Autodesk Fusion 360 part; units mm, degrees
box "Primitiva de caixa1" add length 60 width 30 height 5 placed x (0, 1, 0) y (-1, 0, 0) z (0, 0, 1) at (30, 0, 0)
cylinder "Cilindro primitivo1" cut diameter 10 height -42 placed x (1, 0, 0) y (0, 1, 0) z (0, 0, 1) at (15, 10, 5)
cylinder "Cilindro primitivo2" cut diameter 10 height -21 placed x (1, 0, 0) y (0, 1, 0) z (0, 0, 1) at (15, 50, 5)
cylinder "Cilindro primitivo3" cut diameter 10 height -17 placed x (1, 0, 0) y (0, 1, 0) z (0, 0, 1) at (15, 30, 5)
CAD build for the part. Positions are in the model's coordinates, mm. Give positions to 0.01 mm unless a question says otherwise; leave off trailing zeros. Order: outer loops, then holes, each group sorted by start corner. A loop starts at its lowest first (then second) coordinate and runs counter-clockwise, first axis right, second up. Notation, with made-up numbers: (-22, 15) - (21, 15) arc R16 ccw to (21, 24) - close; hole circle Ø9 at (10.25, 30.25). An arc over 180 degrees is marked (long way). Answer in a Markdown table with one row per item.
1. Probe probe 1 along Y at (x, z) = (15, 2); probe 2 along Y at (x, z) = (17, 1.95); probe 3 along X at (y, z) = (34, 3.25). List the from-to ranges inside material, lowest first. Write a range as [from, to].
Data:
| item | result |
|---|---|
| probe 1 | y = [0, 5], [15, 25], [35, 45], [55, 60] |
| probe 2 | y = [0, 5.42], [14.58, 25.42], [34.58, 45.42], [54.58, 60] |
| probe 3 | x = [0, 12], [18, 30] |
2. Saw through at A-A, the plane y = 10. Give the cut face in (x, z), plus the area to 3 significant figures.
Data:
| item | result |
|---|---|
| outline | (0, 0) - (10, 0) - (10, 5) - (0, 5) - close; (20, 0) - (30, 0) - (30, 5) - (20, 5) - close |
| area | 100 mm² |
3. Saw through at B-B, the plane x = 15. Give the cut face in (y, z).
Data:
| item | result |
|---|---|
| outline | (0, 0) - (5, 0) - (5, 5) - (0, 5) - close; (15, 0) - (25, 0) - (25, 5) - (15, 5) - close; (35, 0) - (45, 0) - (45, 5) - (35, 5) - close; (55, 0) - (60, 0) - (60, 5) - (55, 5) - close |
4. Pull direction X, two halves, no side cores. Call faces 1 (the flat face through (15, 60, 2)), 2 (the flat face through (0, 30, 2)), 3 (the cylindrical face through (18, 54, 3)): pulls with the +X half, pulls with the -X half, needs draft (parallel to the pull), parting line crosses it, or undercut.
Data:
| item | result |
|---|---|
| face 1 | needs draft |
| face 2 | pulls with the -X half |
| face 3 | undercut |
5. Saw through at C-C, the plane z = 2.9. Give the cut face in (x, y).
Data:
| item | result |
|---|---|
| outline | (0, 0) - (30, 0) - (30, 60) - (0, 60) - close; hole circle Ø10 at (15, 10); hole circle Ø10 at (15, 30); hole circle Ø10 at (15, 50) |
